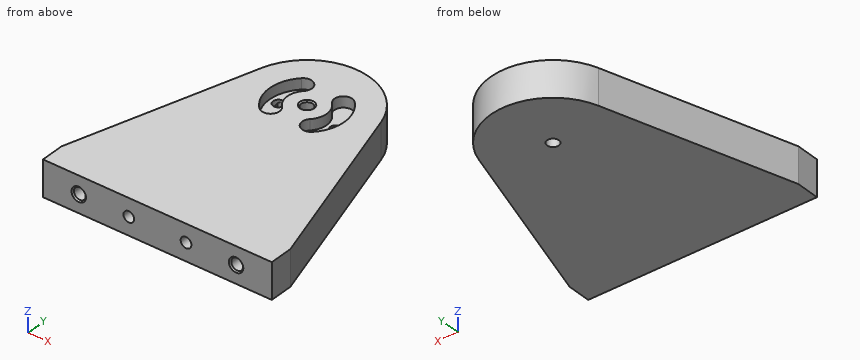
```python
from build123d import *

# Parameters (mm, degrees)
Y_KSEKLIK_EKSTR_ZYON1_DEPTH = 5
M4_DI_LI_DELIK1_D           = 3.3
M4_DI_LI_DELIK1_CSINK_D     = 4.05
M4_DI_LI_DELIK1_CSINK_ANGLE = 90
M4_DI_LI_DELIK2_D           = 3.3
M4_DI_LI_DELIK2_DEPTH       = 12
M4_DI_LI_DELIK2_CSINK_D     = 4.05
M4_DI_LI_DELIK2_CSINK_ANGLE = 90
M4_DI_LI_DELIK2_TIP         = 0.991420021
IZIM12_R                    = 1.5
KES_EKSTR_ZYON1_DEPTH       = 54
KES_EKSTR_ZYON2_DEPTH       = 3
IZIM14_R                    = 1.5
KES_EKSTR_ZYON3_DEPTH       = 5


with BuildPart() as part:
    # Çizim2 → Yükseklik-Ekstrüzyon1 (new, symmetric)
    with BuildSketch(Plane.XY):
        with BuildLine():
            Line((-32, 0), (32, 0))
            Line((32, 0), (32, 6.5))
            Line((32, 6.5), (16.768327291, 57.507314637))
            ThreePointArc((16.768327291, 57.507314637), (0, 70), (-16.768327291, 57.507314637))
            Line((-16.768327291, 57.507314637), (-32, 6.5))
            Line((-32, 6.5), (-32, 0))
        make_face()
    extrude(amount=Y_KSEKLIK_EKSTR_ZYON1_DEPTH, both=True)

    # M4 Dişli Delik1 (through all)
    with Locations(Plane.XY.offset(5)):
        with Locations((0, 52.5)):
            CounterSinkHole(M4_DI_LI_DELIK1_D / 2, M4_DI_LI_DELIK1_CSINK_D / 2, counter_sink_angle=M4_DI_LI_DELIK1_CSINK_ANGLE)

    # M4 Dişli Delik2
    with Locations(Plane(origin=(0, 0, 0), x_dir=(-1, 0, 0), z_dir=(0, -1, 0))):
        with Locations((22, 0), (-22, 0)):
            CounterSinkHole(M4_DI_LI_DELIK2_D / 2, M4_DI_LI_DELIK2_CSINK_D / 2, depth=M4_DI_LI_DELIK2_DEPTH, counter_sink_angle=M4_DI_LI_DELIK2_CSINK_ANGLE)
            with Locations((0, 0, -(M4_DI_LI_DELIK2_DEPTH + M4_DI_LI_DELIK2_TIP / 2))):  # 118° drill point
                Cone(0, M4_DI_LI_DELIK2_D / 2, M4_DI_LI_DELIK2_TIP, mode=Mode.SUBTRACT)

    # Çizim12 → Kes-Ekstrüzyon1 (cut)
    with BuildSketch(Plane.XZ):
        with Locations((-8, 0)):
            Circle(IZIM12_R)
        with Locations((8, 0)):
            Circle(IZIM12_R)
    extrude(amount=-KES_EKSTR_ZYON1_DEPTH, mode=Mode.SUBTRACT)

    # Çizim13 → Kes-Ekstrüzyon2 (cut)
    with BuildSketch(Plane(origin=(0, 0, 5), x_dir=(-1, 0, 0), z_dir=(0, 0, -1))):
        with BuildLine():
            ThreePointArc((7.424621202, 45.075378798), (10.5, 52.5), (7.424621202, 59.924621202))
            ThreePointArc((7.424621202, 59.924621202), (3.889087297, 59.924621202), (3.889087297, 56.389087297))
            ThreePointArc((3.889087297, 56.389087297), (5.5, 52.5), (3.889087297, 48.610912703))
            ThreePointArc((3.889087297, 48.610912703), (3.889087297, 45.075378798), (7.424621202, 45.075378798))
        make_face()
        with BuildLine():
            ThreePointArc((-7.424621202, 45.075378798), (-10.5, 52.5), (-7.424621202, 59.924621202))
            ThreePointArc((-7.424621202, 59.924621202), (-3.889087297, 59.924621202), (-3.889087297, 56.389087297))
            ThreePointArc((-3.889087297, 56.389087297), (-5.5, 52.5), (-3.889087297, 48.610912703))
            ThreePointArc((-3.889087297, 48.610912703), (-3.889087297, 45.075378798), (-7.424621202, 45.075378798))
        make_face()
    extrude(amount=KES_EKSTR_ZYON2_DEPTH, mode=Mode.SUBTRACT)

    # Çizim14 → Kes-Ekstrüzyon3 (cut)
    with BuildSketch(Plane.XY.offset(2)):
        with Locations((-8, 52.5)):
            Circle(IZIM14_R)
        with Locations((8, 52.5)):
            Circle(IZIM14_R)
    extrude(amount=-KES_EKSTR_ZYON3_DEPTH, mode=Mode.SUBTRACT)


solid = part.part
```
The listing builds one solid part. Answer for the finished solid, in the listing's coordinates (mm). Coordinates: 2 decimals unless noted, no trailing zeros. Write each loop counter-clockwise with the first axis right and the second up, starting at its lowest first coordinate (ties: lowest second). Pieces come first, ordered by that corner, then holes.
Q1. Section C-C, the plane y = 59 is taken. Write down the section's boundary in (x, z), then the cut area to 3 significant figures.
Returned:
outline: (-16.25, -5) - (16.25, -5) - (16.25, 5) - (8.25, 5) - (8.25, 2) - (3.3, 2) - (3.3, 5) - (-3.3, 5) - (-3.3, 2) - (-8.25, 2) - (-8.25, 5) - (-16.25, 5) - close
area: 295 mm2
Q2. Given P1, Ø4, axis at y = 48.5, z = 1.5, coming from the +X side; P2, Ø3.5, axis at x = -7.5, y = 53, coming from the +Z side; P3, Ø6, axis at y = 48, z = -1, coming from the +X side; P4, Ø2, axis at x = 0, y = 52.5, coming from the +Z side, each flat-ended and moving along its own axis, determine where each tip first touches the part or whether it passes through.
Returned:
P1: stops at x = 20.06
P2: stops at z = 2
P3: stops at x = 20.5
P4: passes through
Q3. Find the intervals of material crossed by line 1 along X through (y, z) = (52.5, 1.1); line 2 along Y through (x, z) = (0, 0.5); line 3 along X through (y, z) = (33, -1.25), in increasing order.
Returned:
line 1: x = -18.26 to -9.5, -6.5 to -1.65, 1.65 to 6.5, 9.5 to 18.26
line 2: y = 0 to 50.85, 54.15 to 70
line 3: x = -24.09 to -8.83, -7.17 to 7.17, 8.83 to 24.09
Q4. Section D-D, the plane y = 42 is taken. Write down the section's boundary in (x, z), then the cut area to 3 significant figures.
Returned:
outline: (-21.4, -5) - (21.4, -5) - (21.4, 5) - (-21.4, 5) - close; hole circle Ø3 at (-8, 0); hole circle Ø3 at (8, 0)
area: 414 mm2
Q5. Section A-A, the plane y = 10 is taken. Write down the section's boundary in (x, z), then the cut area to 3 significant figures.
Returned:
outline: (-30.95, -5) - (30.95, -5) - (30.95, 5) - (-30.95, 5) - close; hole circle Ø3.3 at (-22, 0); hole circle Ø3 at (-8, 0); hole circle Ø3 at (8, 0); hole circle Ø3.3 at (22, 0)
area: 588 mm2
Q6. Section B-B, the plane y = 20 is taken. Write down the section's boundary in (x, z).
Returned:
outline: (-27.97, -5) - (27.97, -5) - (27.97, 5) - (-27.97, 5) - close; hole circle Ø3 at (-8, 0); hole circle Ø3 at (8, 0)
